```python
from build123d import *

# Parameters (mm, degrees)
F1_DEPTH    = 25
F2_W        = 37
F2_H        = 0.8
F3_DEPTH    = 10
F4_W        = 37
F4_H        = 0.8
F5_DEPTH    = 10
F6_T        = 0.8
F6_T3_DEPTH = 26.6
F6_T5_DEPTH = 38.6
F9_DEPTH    = 2


# Not quite as in the source:
# - a shell that OpenCascade refuses in one call is made with other operations: the cavity is built on its own and cut out


with BuildPart() as f1:
    # F0 (on Top) → F1 (new body)
    with BuildSketch(Plane.XY):
        Polygon((-33.6095448622, 23.5), (-33.6095448622, -23.5), (-24.6095448622, -23.5), (-24.6095448622, -35), (12.3904551378, -35), (12.3904551378, -23.5), (21.3904551378, -23.5), (21.3904551378, 23.5), (12.3904551378, 23.5), (12.3904551378, 35), (-24.6095448622, 35), (-24.6095448622, 23.5), align=None)
    extrude(amount=F1_DEPTH)

    # F2 (on face) → F3 (join)
    with BuildSketch(Plane.XZ.offset(35)):
        with Locations((-6.1095448622, 0.4)):
            Rectangle(F2_W, F2_H)
    extrude(amount=F3_DEPTH)

    # F4 (on face) → F5 (join)
    with BuildSketch(Plane(origin=(0, 35, 0), x_dir=(-1, 0, 0), z_dir=(0, 1, 0))):
        with Locations((6.1095448622, 0.4)):
            Rectangle(F4_W, F4_H)
    extrude(amount=F5_DEPTH)

    # F6: shell of thickness 0.8, made by hand


with BuildPart() as f6_core1:
    # F6_t2: copy of F1
    add(f1.part)

    # the walls: a layer under each face that stays
    f6_faces = [f6_core1.faces().sort_by_distance(p)[0] for p in [
        (-33.6095448622, 0, 12.5),
        (-6.1095448622, 0, 25),
        (-24.6095448622, 34.25, 12.5),
        (-6.1095448622, 40, 0.8),
        (-6.1095448622, 45, 0.4),
        (-6.1095448622, 35, 12.9),
        (12.3904551378, 34.25, 12.5),
        (16.8904551378, 23.5, 12.5),
        (21.3904551378, 0, 12.5),
        (16.8904551378, -23.5, 12.5),
        (12.3904551378, -34.25, 12.5),
        (-6.1095448622, -40, 0.8),
        (-6.1095448622, -45, 0.4),
        (-6.1095448622, -35, 12.9),
        (-24.6095448622, -34.25, 12.5),
        (-29.1095448622, -23.5, 12.5),
        (-29.1095448622, 23.5, 12.5),
    ]]
    thicken(f6_faces, amount=-F6_T, mode=Mode.SUBTRACT)

    # F6_s4 → F6_t3 (cut)
    with BuildSketch(Plane.XY.offset(-0.8)):
        Polygon((-24.6175448622, 23.508), (-23.8095448622, 23.5), (-23.8095448622, 22.7), (-24.6095448622, 22.7), align=None)
        Polygon((12.3984551378, 23.508), (11.5904551378, 23.5), (11.5904551378, 22.7), (12.3904551378, 22.7), align=None)
        Polygon((12.3984551378, -23.508), (12.3904551378, -22.7), (11.5904551378, -22.7), (11.5904551378, -23.5), align=None)
        Polygon((-24.6175448622, -23.508), (-23.8095448622, -23.5), (-23.8095448622, -22.7), (-24.6095448622, -22.7), align=None)
    extrude(amount=F6_T3_DEPTH, mode=Mode.SUBTRACT)

    # F6_s6 → F6_t5 (cut)
    with BuildSketch(Plane.YZ.offset(-25.4095448622)):
        Polygon((35.008, 0.808), (35, 0), (34.2, 0), (34.2, 0.8), align=None)
        Polygon((-35.008, 0.808), (-35, 0), (-34.2, 0), (-34.2, 0.8), align=None)
    extrude(amount=F6_T5_DEPTH, mode=Mode.SUBTRACT)


with BuildPart() as f1_1:
    add(f1.part)

    # what is left inside the walls is the cavity
    f6_cavity = [f6_core1.part.solids().sort_by_distance(p)[0] for p in [
        (-6.109545, -11.4, 24.192),
    ]]
    add(f6_cavity, mode=Mode.SUBTRACT)

    # F8 (on face) + F7 (on face) → F9 (cut)
    with BuildSketch(Plane.XY.offset(0.8)):
        with BuildLine():
            Line((-8.6095448622, -37.5000002948), (-8.6095448622, -45))
            Line((-8.6095448622, -45), (-3.6095448622, -45))
            Line((-3.6095448622, -45), (-3.6095448622, -37.5))
            ThreePointArc((-3.6095448622, -37.5), (-4.3417779216, -35.7322330347), (-6.1095448972, -35))
            ThreePointArc((-6.1095448972, -35), (-7.8773119318, -35.7322331636), (-8.6095448622, -37.5000002948))
        make_face()
    with BuildSketch(Plane.XY.offset(0.8)):
        with BuildLine():
            Line((-3.6095448622, 37.5), (-3.6095448622, 45))
            Line((-3.6095448622, 45), (-8.6095448622, 45))
            Line((-8.6095448622, 45), (-8.6095448622, 37.5))
            ThreePointArc((-8.6095448622, 37.5), (-7.8773118305, 35.7322330623), (-6.1095449054, 35))
            ThreePointArc((-6.1095449054, 35), (-4.3417779245, 35.7322330318), (-3.6095448622, 37.5))
        make_face()
    extrude(amount=-F9_DEPTH, mode=Mode.SUBTRACT)


solid = f1_1.part
```
Can you work these out from the model? Positions are in its coordinate system, mm. A direction names the side the tool comes from. Give positions to 0.01 mm unless a question says otherwise; leave off trailing zeros. Order: outer loops, then holes, each group sorted by start corner. A loop starts at its lowest first (then second) coordinate and runs counter-clockwise, first axis right, second up. Notation, with made-up numbers: M 52.5,-31.5 L 57.5,-31.5 A17 ccw 57.5,-15.5 Z; hole C 56.5,1.25 d9. An arc over 180 degrees is marked long. Write item = value, one per line. Start each with the question number.
Q1. I need wall thicknesses on probe 1 along X at (y, z) = (32, 10); probe 2 along X at (y, z) = (-10.5, 23); probe 3 along Y at (x, z) = (-26.5, 21.5). Which ranges of each line are inside material? Lowest first, please. Write a range as [from, to].
Q2. We'd pull the mould along Y, two halves only. Please class faces 6 (the flat face through (-23.81, 29, 12)), 7 (the flat face through (-6, -35, 13)), 8 (the flat face through (-18, -40, 0.8)): pulls with the +Y half, pulls with the -Y half, needs draft (parallel to the pull), parting line crosses it, or undercut.
Q3. Suppose I cut it at C-C (x = 13.5). Write out the boundary of the cut face in (y, z).
Q4. Suppose I cut it at B-B (z = 6.75). Write out the boundary of the cut face in (x, y).
Q5. Will these pins go through, and if not, where does the flat tip stop? pin 1 Ø1 at (x, z) = (-10.5, 10.5) entering from +Y; pin 2 Ø11 at (y, z) = (37, 9) entering from -X; pin 3 Ø6 at (x, z) = (-15, 3) entering from +Y; pin 4 Ø16 at (x, y) = (-14.5, -4) entering from -Z.
Q6. Suppose I cut it at D-D (y = 2). Write out the boundary of the cut face in (x, z).
Q7. Suppose I cut it at A-A (y = -39). Write out the boundary of the cut face in (x, z), plus the area to 3 significant figures.
Q8. For faces 1 (the flat face through (5, 40, 0.8)), 2 (the flat face through (12.39, -29, 12)), 3 (the flat face through (-24.61, 29, 12)), 4 (the flat face through (3, -40, 0.8)), 5 (the flat face through (-28, -22.7, 12)), which set-ups out of +Z, -Z, +X, -X, +Y, -Y let a thin tool reach every point of the face, with its end or its side?
Check result:
q1.probe_1 = [-24.61, -23.81], [11.59, 12.39]
q1.probe_2 = [-33.61, -32.81], [20.59, 21.39]
q1.probe_3 = [-23.5, -22.7], [22.7, 23.5]
q2.face_6 = undercut
q2.face_7 = pulls with the -Y half
q2.face_8 = needs draft
q3.outline = M -23.5,0 L -22.7,0 L -22.7,24.2 L 22.7,24.2 L 22.7,0 L 23.5,0 L 23.5,25 L -23.5,25 Z
q4.outline = M -33.61,-23.5 L -24.61,-23.5 L -24.61,-35 L 12.39,-35 L 12.39,-23.5 L 21.39,-23.5 L 21.39,23.5 L 12.39,23.5 L 12.39,35 L -24.61,35 L -24.61,23.5 L -33.61,23.5 Z; hole M -32.81,-22.7 L -23.81,-22.7 L -23.81,-34.2 L 11.59,-34.2 L 11.59,-22.7 L 20.59,-22.7 L 20.59,22.7 L 11.59,22.7 L 11.59,34.2 L -23.81,34.2 L -23.81,22.7 L -32.81,22.7 Z
q5.pin_1 = 35
q5.pin_2 = -24.61
q5.pin_3 = 45
q5.pin_4 = 24.2
q6.outline = M -33.61,0 L -32.81,0 L -32.81,24.2 L 20.59,24.2 L 20.59,0 L 21.39,0 L 21.39,25 L -33.61,25 Z
q7.outline = M -24.61,0 L -8.61,0 L -8.61,0.8 L -24.61,0.8 Z; M -3.61,0 L 12.39,0 L 12.39,0.8 L -3.61,0.8 Z
q7.area = 25.6 mm2
q8.face_1 = +Z, +X, -X, +Y
q8.face_2 = +Z, -Z, +X, -Y
q8.face_3 = +Z, -Z, -X, +Y
q8.face_4 = +Z, +X, -X, -Y
q8.face_5 = -Z
